Here's how the part is built. I have some questions about the finished solid (model axes, mm). A direction names the side the tool comes from. Round coordinates to 2 decimals unless told otherwise and drop trailing zeros. Write each loop counter-clockwise with the first axis right and the second up, starting at its lowest first coordinate (ties: lowest second). Pieces come first, ordered by that corner, then holes. Notation, with made-up numbers: (28, 61) - (69, 61) arc R29 ccw to (69, 93) - close; hole circle Ø10 at (46.25, 24). An arc over 180 degrees is marked (long way). One line per item, written item: value. Start each with the question number.
Item 1: For P1, Ø3, axis at x = 18, y = 3.5, coming from the -Z side; P2, Ø8, axis at x = 3.5, y = -7.5, coming from the -Z side; P3, Ø1, axis at x = 7, z = -2.5, coming from the -Y side, each with a flat end and sliding along its axis, tell me the tip position at first contact or that it passes through.
Item 2: Imagine slicing it at D-D, the plane x = 19.05. Please give me the cut outline in (y, z) (3 decimals), then the cut area to 3 significant figures.
Item 3: Imagine slicing it at B-B, the plane x = 15.75. Please give me the cut outline in (y, z) (3 decimals).
Item 4: Imagine slicing it at A-A, the plane z = 0. Please give me the cut outline in (x, y) (3 decimals), then the cut area to 3 significant figures.
Item 5: For faces 1 (the face through (0, 3, 0)), 2 (the face through (25.4, -13, 0)), 3 (the face through (12.7, 2, 3)), 4 (the face through (19, 0, -11.773)), 5 (the face through (19, 11.773, 0)), which set-ups out of +Z, -Z, +X, -X, +Y, -Y let a thin tool reach every point of the face, with its end or its side?
Item 6: Imagine slicing it at C-C, the plane y = 0. Please give me the cut outline in (x, z) (3 decimals).
Item 7: Thinking about a two-plate mould opening in Z: for faces 6 (the face through (12.52, 7.33, -14.08)), 7 (the face through (1.211, -1.451, -1.113)), 8 (the face through (20.34, -0.41, 13.8)), 9 (the face through (21, 0, 11.773)), which applies, released by +Z, released by -Z, zero draft, split by the parting line, or undercut?
Item 8: If I drill on line 1 (Z direction, x = 6.5, y = 0) (3 decimals); line 2 (X direction, y = 0, z = 14.9); line 3 (Z direction, x = 1.05, y = 0) (3 decimals), over which ranges is the centre line in solid material (lowest first)?
```python
from build123d import *

# Parameters (mm, degrees)
F0_R     = 15.875
F1_DEPTH = 25.4
F2_W     = 23.5458
F2_H     = 23.5458
F3_DEPTH = 12.7
F4_R     = 3.175
F5_DEPTH = 23.0124
F6_R     = 1.8288
F7_DEPTH = 12.701
F8_R     = 1.35255
F9_DEPTH = 4.1031


with BuildPart() as f1:
    # F0 (on Right) → F1 (new body)
    with BuildSketch(Plane.YZ):
        Circle(F0_R)
    extrude(amount=F1_DEPTH)

    # F2 (on face) → F3 (cut)
    with BuildSketch(Plane.YZ.offset(25.4)):
        Rectangle(F2_W, F2_H)
    extrude(amount=-F3_DEPTH, mode=Mode.SUBTRACT)

    # F4 (on face) → F5 (cut)
    with BuildSketch(Plane.YZ.offset(25.4)):
        Circle(F4_R)
    extrude(amount=-F5_DEPTH, mode=Mode.SUBTRACT)

    # F6 (on face) → F7 (cut, through all)
    with BuildSketch(Plane.YZ.offset(12.7)):
        Circle(F6_R)
    extrude(amount=-F7_DEPTH, mode=Mode.SUBTRACT)

    # F8 (on face) → F9 (cut, through all)
    with BuildSketch(Plane(origin=(0, 0, 11.7729), x_dir=(1, 0, 0), z_dir=(0, 0, -1))):
        with Locations((19.05, 0)):
            Circle(F8_R)
    extrude(amount=-F9_DEPTH, mode=Mode.SUBTRACT)


solid = f1.part
```
Values follow:
1. P1: stops at z = -15.75
1. P2: stops at z = -15.48
1. P3: stops at y = -15.75
2. outline: (-11.773, -10.65) - (-11.773, 10.65) arc R15.875 ccw to start; (-10.65, -11.773) arc R15.875 ccw to (10.65, -11.773) - close; (-10.65, 11.773) - (-1.353, 11.773) - (-1.353, 15.817) arc R15.875 ccw to start; (1.353, 11.773) - (10.65, 11.773) arc R15.875 ccw to (1.353, 15.817) - close; (11.773, -10.65) arc R15.875 ccw to (11.773, 10.65) - close
2. area: 229 mm^2
3. outline: (-11.773, -10.65) - (-11.773, 10.65) arc R15.875 ccw to start; (-10.65, -11.773) arc R15.875 ccw to (10.65, -11.773) - close; (-10.65, 11.773) - (10.65, 11.773) arc R15.875 ccw to start; (11.773, -10.65) arc R15.875 ccw to (11.773, 10.65) - close
4. outline: (0, -15.875) - (25.4, -15.875) - (25.4, -11.773) - (12.7, -11.773) - (12.7, -3.175) - (2.388, -3.175) - (2.388, -1.829) - (0, -1.829) - close; (0, 1.829) - (2.388, 1.829) - (2.388, 3.175) - (12.7, 3.175) - (12.7, 11.773) - (25.4, 11.773) - (25.4, 15.875) - (0, 15.875) - close
4. area: 433 mm^2
5. face 1: +Z, -Z, -X, +Y, -Y
5. face 2: +Z, -Z, +X, +Y, -Y
5. face 3: +X
5. face 4: +X, +Y, -Y
5. face 5: +Z, -Z, +X
6. outline: (0, -15.875) - (25.4, -15.875) - (25.4, -11.773) - (12.7, -11.773) - (12.7, -3.175) - (2.388, -3.175) - (2.388, -1.829) - (0, -1.829) - close; (0, 1.829) - (2.388, 1.829) - (2.388, 3.175) - (12.7, 3.175) - (12.7, 11.773) - (17.697, 11.773) - (17.697, 15.875) - (0, 15.875) - close; (20.403, 11.773) - (25.4, 11.773) - (25.4, 15.875) - (20.403, 15.875) - close
7. face 6: split by the parting line
7. face 7: undercut
7. face 8: zero draft
7. face 9: undercut
8. line 1: z = -15.875 to -3.175, 3.175 to 15.875
8. line 2: x = 0 to 17.7, 20.4 to 25.4
8. line 3: z = -15.875 to -1.829, 1.829 to 15.875
